from build123d import *

# Parameters (mm, degrees)
SKETCH1_W                 = 3
SKETCH1_H                 = 15
BOSS_EXTRUDE1_DEPTH       = 25
SKETCH2_W                 = 25
SKETCH2_H                 = 10
BOSS_EXTRUDE2_DEPTH       = 6
FILLET1_SIZE              = 3
FILLET1_SIZE_2            = 5
F_3_0MM_DOWEL_HOLE1_D     = 3
F_3_0MM_DOWEL_HOLE1_DEPTH = 5
F_3_0MM_DOWEL_HOLE1_TIP   = 0.901290929
SKETCH5_W                 = 11.909967374
SKETCH5_H                 = 2.030245184
CUT_EXTRUDE1_DEPTH        = 18


with BuildPart() as part:
    # Sketch1 → Boss-Extrude1 (new body)
    with BuildSketch(Plane(origin=(0, 0, 0), x_dir=(0, 0, -1), z_dir=(1, 0, 0))):
        with Locations((1.5, 7.5)):
            Rectangle(SKETCH1_W, SKETCH1_H)
    extrude(amount=BOSS_EXTRUDE1_DEPTH)

    # Sketch2 → Boss-Extrude2 (add)
    with BuildSketch(Plane(origin=(0, 0, -3), x_dir=(-1, 0, 0), z_dir=(0, 0, -1))):
        with Locations((-12.5, 10)):
            Rectangle(SKETCH2_W, SKETCH2_H)
    extrude(amount=BOSS_EXTRUDE2_DEPTH)

    # Fillet1
    # an asymmetric fillet: 5, 3 mm, written as the material it takes off along each edge
    with BuildSketch(Plane(origin=(-12.5, 15, 0), x_dir=(0, 0, -1), z_dir=(1, 0, 0))) as fillet1_piece_1:
        with BuildLine():
            Bezier((FILLET1_SIZE, 0), (0, 0), (0, -FILLET1_SIZE_2), weights=[1, 0.707106781, 1])
            Line((0, -FILLET1_SIZE_2), (0, 0))
            Line((0, 0), (FILLET1_SIZE, 0))
        make_face()
    extrude(amount=50, mode=Mode.SUBTRACT)

    # Ø3.0mm Dowel Hole1
    with Locations(Plane(origin=(0, 5, 0), x_dir=(-1, 0, 0), z_dir=(0, -1, 0))):
        with Locations((-3, 6), (-18, 6), (-7, 6), (-22, 6)):
            Hole(F_3_0MM_DOWEL_HOLE1_D / 2, depth=F_3_0MM_DOWEL_HOLE1_DEPTH)
            with Locations((0, 0, -(F_3_0MM_DOWEL_HOLE1_DEPTH + F_3_0MM_DOWEL_HOLE1_TIP / 2))):  # 118° drill point
                Cone(0, F_3_0MM_DOWEL_HOLE1_D / 2, F_3_0MM_DOWEL_HOLE1_TIP, mode=Mode.SUBTRACT)

    # Sketch5 → Cut-Extrude1 (cut)
    with BuildSketch(Plane(origin=(0, 15, 0), x_dir=(1, 0, 0), z_dir=(0, 1, 0))):
        with Locations((12.749835557, -0.102167309)):
            Rectangle(SKETCH5_W, SKETCH5_H)
    extrude(amount=-CUT_EXTRUDE1_DEPTH, mode=Mode.SUBTRACT)


solid = part.part
CAD build for the part. Positions are in the model's coordinates, mm. A direction names the side the tool comes from. Give positions to 0.01 mm unless a question says otherwise; leave off trailing zeros. Order: outer loops, then holes, each group sorted by start corner. A loop starts at its lowest first (then second) coordinate and runs counter-clockwise, first axis right, second up. Notation, with made-up numbers: (-19.5, -32) -> (-8.5, -32) arc R17 ccw to (-8.5, -7) -> close; hole circle Ø1 at (15, 89.25). An arc over 180 degrees is marked (long way). Return JSON: item names as keys, results as strings.
Q1. Drill centre lines: line 1 (X direction, y = 6.6, z = -6); line 2 (X direction, y = 6.5, z = -0.75); line 3 (Z direction, x = 22, y = 6.4). Where is each one in solid material? Low to high.
Working result:
{"line 1": "0 to 1.5, 4.5 to 5.5, 8.5 to 16.5, 19.5 to 20.5, 23.5 to 25", "line 2": "0 to 6.79, 18.7 to 25", "line 3": "-9 to -7.5, -4.5 to 0"}
Q2. Flat gauge pins, fed straight in: pin 1 (3 mm diameter, centred on x = 10, z = -7, fed in from -Y); pin 2 (3 mm diameter, centred on x = 15.5, y = 9, fed in from +Z); pin 3 (5.5 mm diameter, centred on x = 16, y = 2, fed in from -Z). Where does each tip first touch, or does it go through?
Working result:
{"pin 1": "y = 5", "pin 2": "z = -0.91", "pin 3": "z = -3"}
Q3. Saw through at A-A (y = 6.5). Write the cut outline in (x, z).
Working result:
{"outline": "(0, -9) -> (25, -9) -> (25, 0) -> (18.7, 0) -> (18.7, -0.91) -> (6.79, -0.91) -> (6.79, 0) -> (0, 0) -> close; hole circle Ø3 at (3, -6); hole circle Ø3 at (7, -6); hole circle Ø3 at (18, -6); hole circle Ø3 at (22, -6)"}
Q4. Saw through at B-B (z = -4.25). Write the cut outline in (x, y).
Working result:
{"outline": "(0, 5) -> (25, 5) -> (25, 15) -> (0, 15) -> close"}
Q5. Mould opens along Z. For faces 1 (the face through (13, 7, -0.913)), 2 (the face through (0, 9, -4)), 3 (the face through (21.759, 10.745, -5.9)) say: pulls with the +Z half, pulls with the -Z half, needs draft (parallel to the pull), parting line crosses it, or undercut.
Working result:
{"face 1": "pulls with the +Z half", "face 2": "needs draft", "face 3": "undercut"}
Q6. Which spindle directions (+Z, -Z, +X, -X, +Y, -Y) get a long thin tool onto all of the face, cutting with end or side? Do faces 4 (the face through (16.5, 7.54, -6.07)), 5 (the face through (25, 9, -4)), 6 (the face through (22, 5, 0)), 7 (the face through (13, 5, -6)), 8 (the face through (18.705, 6.9, -0.5)). Say none if no direction does.
Working result:
{"face 4": "-Y", "face 5": "+Z, -Z, +X, +Y, -Y", "face 6": "+Z, +X, -X, +Y, -Y", "face 7": "-Z, +X, -X, -Y", "face 8": "+Z, +Y, -Y"}
